The model under review builds one solid part; all positions refer to its coordinate system, in mm. Face numbers are marked on the shaded views. A direction names the side the tool comes from. Give positions to 0.01 mm unless a question says otherwise; leave off trailing zeros. Order: outer loops, then holes, each group sorted by start corner. A loop starts at its lowest first (then second) coordinate and runs counter-clockwise, first axis right, second up.
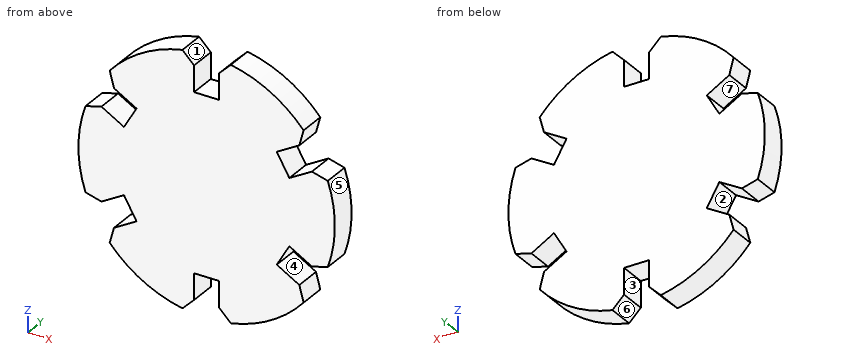
```python
from build123d import *

# Parameters (mm, degrees)
SKETCH1_R           = 25
BOSS_EXTRUDE1_DEPTH = 5.2
SKETCH2_W           = 4.9
SKETCH2_H           = 7.8
CUT_EXTRUDE1_DEPTH  = 5.2
CHAMFER1_SIZE       = 2.6


with BuildPart() as part:
    # Sketch1 → Boss-Extrude1 (new body)
    with BuildSketch(Plane(origin=(0, 0, 0), x_dir=(1, 0, 0), z_dir=(0, 1, 0))):
        with Locations(Location((0, 0, 0), (0, 0, 270))):
            Circle(SKETCH1_R)
    extrude(amount=BOSS_EXTRUDE1_DEPTH)

    # Sketch2 → Cut-Extrude1 (cut)
    with BuildSketch(Plane(origin=(0, 5.2, 0), x_dir=(1, 0, 0), z_dir=(0, 1, 0))):
        Polygon((22.875635095, 10.378237761), (16.120636945, 6.478237761), (13.670636945, 10.721762239), (20.425635095, 14.621762239), align=None)
        with Locations((0, 21.1)):
            Rectangle(SKETCH2_W, SKETCH2_H)
        Polygon((20.425635095, -14.621762239), (13.670636945, -10.721762239), (16.120636945, -6.478237761), (22.875635095, -10.378237761), align=None)
        with Locations((0, -21.1)):
            Rectangle(SKETCH2_W, SKETCH2_H)
        Polygon((-22.875635095, -10.378237761), (-16.120636945, -6.478237761), (-13.670636945, -10.721762239), (-20.425635095, -14.621762239), align=None)
        Polygon((-20.425635095, 14.621762239), (-13.670636945, 10.721762239), (-16.120636945, 6.478237761), (-22.875635095, 10.378237761), align=None)
    extrude(amount=-CUT_EXTRUDE1_DEPTH, mode=Mode.SUBTRACT)

    # Chamfer1
    # the kernel refuses this chamfer: 2.6, 2.378368378 mm, written as the material it takes off along each edge
    with BuildSketch(Plane(origin=(20.321417916, 11.886375769, -14.561592423), x_dir=(-0.6191501526996462, 0, -0.7852726204395546), z_dir=(0, -1, 0)), Plane(origin=(-2.45, 11.886375769, -24.879660367), x_dir=(-0.9896411145468598, 0, 0.14356345077508154), z_dir=(0, -1, 0)), Plane(origin=(-22.771417916, 11.886375769, -10.318067944), x_dir=(-0.37049096184717384, 0, 0.9288360712146981), z_dir=(0, -1, 0)), Plane(origin=(-20.321417916, 11.886375769, 14.561592423), x_dir=(0.6191501526997778, 0, 0.785272620439451), z_dir=(0, -1, 0)), Plane(origin=(2.45, 11.886375769, 24.879660367), x_dir=(0.9896411145468216, 0, -0.14356345077534402), z_dir=(0, -1, 0)), Plane(origin=(22.771417916, 11.886375769, 10.318067944), x_dir=(0.3704909618470835, 0, -0.9288360712147342), z_dir=(0, -1, 0))) as chamfer1_piece_1:
        with BuildLine():
            Line((2.294378332, 0), (CHAMFER1_SIZE * 0.143563450775, -CHAMFER1_SIZE * 0.989641114547))
            Line((CHAMFER1_SIZE * 0.143563450775, -CHAMFER1_SIZE * 0.989641114547), (0, 0))
            ThreePointArc((0, 0), (1.178279971, 0.026315397), (2.294378332, 0))
        make_face()
    extrude(amount=18.572751537, mode=Mode.SUBTRACT)
    with BuildSketch(Plane(origin=(22.771417916, 11.886375769, -10.318067944), x_dir=(-0.8660254037844386, 0, 0.49999999999999983), z_dir=(0, -1, 0)), Plane(origin=(2.45, 11.886375769, -24.879660367), x_dir=(0, 0, 1), z_dir=(0, -1, 0)), Plane(origin=(-20.321417916, 11.886375769, -14.561592423), x_dir=(0.8660254037844397, 0, 0.4999999999999983), z_dir=(0, -1, 0)), Plane(origin=(-22.771417916, 11.886375769, 10.318067944), x_dir=(0.8660254037844377, 0, -0.5000000000000014), z_dir=(0, -1, 0)), Plane(origin=(-2.45, 11.886375769, 24.879660367), x_dir=(0, 0, -1), z_dir=(0, -1, 0))) as chamfer1_piece_2:
        with BuildLine():
            Line((CHAMFER1_SIZE, 0), (0.329388871, -2.270611129))
            ThreePointArc((0.329388871, -2.270611129), (0.14311514, -1.169852233), (0, 0))
            Line((0, 0), (CHAMFER1_SIZE, 0))
        make_face()
    extrude(amount=18.572751537, mode=Mode.SUBTRACT)
    with BuildSketch(Plane(origin=(20.321417916, 11.886375769, 14.561592423), x_dir=(-0.6191501526994649, 0, 0.7852726204396976), z_dir=(0, -1, 0))) as chamfer1_piece_3:
        with BuildLine():
            Line((2.294378332, 0), (CHAMFER1_SIZE * 0.143563450775, CHAMFER1_SIZE * 0.989641114547))
            Line((CHAMFER1_SIZE * 0.143563450775, CHAMFER1_SIZE * 0.989641114547), (0, 0))
            ThreePointArc((0, 0), (1.178279971, -0.026315397), (2.294378332, 0))
        make_face()
    extrude(amount=18.572751537, mode=Mode.SUBTRACT)


solid = part.part
```
Item 1: Take a section at C-C (z = -4.5). Give the boundary of the cut face in (x, y).
Values found:
outline: (-24.59, 0) - (24.59, 0) - (24.59, 5.2) - (-24.59, 5.2) - close
Item 2: Take a section at B-B (x = -12). Give the boundary of the cut face in (y, z), and give its area (3 significant figures).
Values found:
outline: (0, -21.93) - (5.2, -21.93) - (5.2, 21.93) - (0, 21.93) - close
area: 228 mm2
Item 3: Clearance check with flat-ended pins moving along their axes: pin 1 Ø2 at (y, z) = (1.5, 14.5) entering from +X; pin 2 Ø1.5 at (x, y) = (-1, 3) entering from +Z; pin 3 Ø2.5 at (y, z) = (3.5, 19.5) entering from +X. State where each tip first meets the part, or that it passes through.
Values found:
pin 1: stops at x = 18.67
pin 2: stops at z = 17.2
pin 3: stops at x = 17.09
Item 4: Draft analysis for pull direction Z (two halves, no side actions). For the marked faces 5, 6 and 7, state which applies: released by +Z, released by -Z, zero draft, split by the parting line, or undercut.
Values found:
face 5: split by the parting line
face 6: released by -Z
face 7: undercut
Item 5: For the marked faces 1, 2, 3 and 4, list the 3-axis set-ups (+Z, -Z, +X, -X, +Y, -Y) from which the entire face can be reached by the end or side of a thin tool; tool diameter is ignored.
Values found:
face 1: +Z, +Y, -Y
face 2: +Y, -Y
face 3: -Z, +Y, -Y
face 4: +X, +Y, -Y
Item 6: Take a section at A-A (z = 20). Give the boundary of the cut face in (x, y), and give its area (3 significant figures).
Values found:
outline: (-15, 0) - (-2.45, 0) - (-2.45, 5.2) - (-15, 5.2) - close; (2.45, 0) - (15, 0) - (15, 5.2) - (2.45, 5.2) - close
area: 131 mm2
Item 7: For line 1 (Z direction, x = 17.5, y = 2.4); line 2 (X direction, y = 0.3, z = 22); line 3 (X direction, y = 4.05, z = 18), list the stretches that pass through material, from the lowest coordinate up.
Values found:
line 1: z = -17.85 to -12.93, -7.27 to 7.27, 12.93 to 17.85
line 2: x = -11.87 to -2.45, 2.45 to 11.87
line 3: x = -17.35 to -2.45, 2.45 to 17.35
